Could you check a few things on this model? Use its own coordinates, in mm. Round coordinates to 2 decimals unless told otherwise and drop trailing zeros. Order: outer loops, then holes, each group sorted by start corner. A loop starts at its lowest first (then second) coordinate and runs counter-clockwise, first axis right, second up. Notation, with made-up numbers: (88, -19) -> (139, -19) arc R29 ccw to (139, 16) -> close; hole circle Ø8 at (45.25, 12). An arc over 180 degrees is marked (long way). Put each result on its own line as item: value. Start each with the question number.
from build123d import *

# Parameters (mm, degrees)
SKETCH1_W           = 609.6
SKETCH1_H           = 1219.2
BOSS_EXTRUDE1_DEPTH = 12.7
SKETCH6_R           = 31.75
CUT_EXTRUDE3_DEPTH  = 682.671834536
SKETCH8_W           = 415.926094716
SKETCH8_H           = 177.8
CUT_EXTRUDE4_DEPTH  = 682.671834536
SKETCH10_W          = 180.418217341
SKETCH10_H          = 88.9
CUT_EXTRUDE7_DEPTH  = 682.671834536
SKETCH14_R          = 44.45
CUT_EXTRUDE8_DEPTH  = 682.671834536


with BuildPart() as part:
    # Sketch1 → Boss-Extrude1 (new body)
    with BuildSketch(Plane(origin=(0, 0, 0), x_dir=(1, 0, 0), z_dir=(0, 1, 0))):
        Rectangle(SKETCH1_W, SKETCH1_H)
    extrude(amount=BOSS_EXTRUDE1_DEPTH)

    # Sketch6 → Cut-Extrude3 (cut, through all)
    with BuildSketch(Plane(origin=(0, 12.7, 0), x_dir=(-1, 0, 0), z_dir=(0, 1, 0))):
        with Locations(Location((0, 0, 0), (0, 0, 90))):
            Circle(SKETCH6_R)
    extrude(amount=-CUT_EXTRUDE3_DEPTH, mode=Mode.SUBTRACT)

    # Sketch8 → Cut-Extrude4 (cut, through all)
    with BuildSketch(Plane(origin=(0, 12.7, 0), x_dir=(1, 0, 0), z_dir=(0, 1, 0))):
        with Locations((461.963047358, 0)):
            Rectangle(SKETCH8_W, SKETCH8_H)
    extrude(amount=-CUT_EXTRUDE4_DEPTH, mode=Mode.SUBTRACT)

    # Sketch10 → Cut-Extrude7 (cut, through all)
    with BuildSketch(Plane(origin=(0, 12.7, 0), x_dir=(1, 0, 0), z_dir=(0, 1, 0))):
        with Locations((-318.80910867, 0)):
            Rectangle(SKETCH10_W, SKETCH10_H)
    extrude(amount=-CUT_EXTRUDE7_DEPTH, mode=Mode.SUBTRACT)

    # Sketch14 → Cut-Extrude8 (cut, through all)
    with BuildSketch(Plane(origin=(0, 12.7, 0), x_dir=(1, 0, 0), z_dir=(0, 1, 0))):
        with Locations((-228.6, 0)):
            Circle(SKETCH14_R)
    extrude(amount=-CUT_EXTRUDE8_DEPTH, mode=Mode.SUBTRACT)


solid = part.part
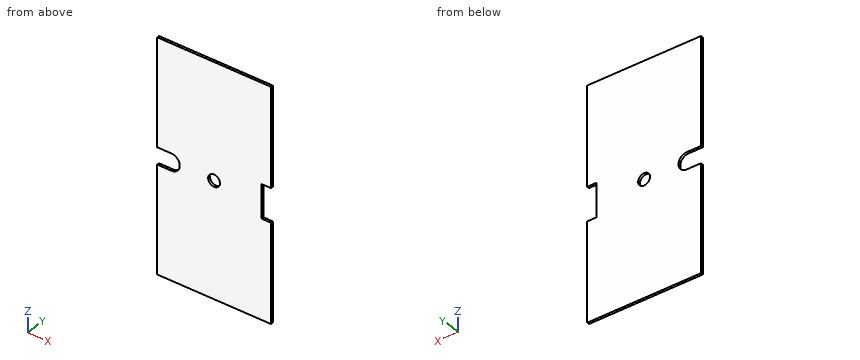
1. I need wall thicknesses on L1, parallel to X at y = 8.25, z = 0; L2, parallel to Z at x = -232, y = 2.5; L3, parallel to X at y = 10.25, z = -50. Which ranges of each line are inside material? Lowest first, please.
2. If we section it at B-B, the plane y = 6.5: Please give me the cut outline in (x, z).
3. For pin 1 Ø6.5 at (y, z) = (6, 19) entering from +X, with a flat end and sliding along its axis, tell me the tip position at first contact or that it passes through.
4. If we section it at A-A, the plane z = 0: Please give me the cut outline in (x, y).
5. If we section it at C-C, the plane x = 0: Please give me the cut outline in (y, z), then the cut area to 3 significant figures.
Results below:
1. L1: -184.15 to -31.75, 31.75 to 254
1. L2: -609.6 to -44.45, 44.45 to 609.6
1. L3: -304.8 to 254
2. outline: (-304.8, -609.6) -> (304.8, -609.6) -> (304.8, -88.9) -> (254, -88.9) -> (254, 88.9) -> (304.8, 88.9) -> (304.8, 609.6) -> (-304.8, 609.6) -> (-304.8, 44.45) -> (-228.6, 44.45) arc R44.45 cw to (-228.6, -44.45) -> (-304.8, -44.45) -> close; hole circle Ø63.5 at (0, 0)
3. pin 1: x = 254
4. outline: (-184.15, 0) -> (-31.75, 0) -> (-31.75, 12.7) -> (-184.15, 12.7) -> close; (31.75, 0) -> (254, 0) -> (254, 12.7) -> (31.75, 12.7) -> close
5. outline: (0, -609.6) -> (12.7, -609.6) -> (12.7, -31.75) -> (0, -31.75) -> close; (0, 31.75) -> (12.7, 31.75) -> (12.7, 609.6) -> (0, 609.6) -> close
5. area: 14,700 mm2
